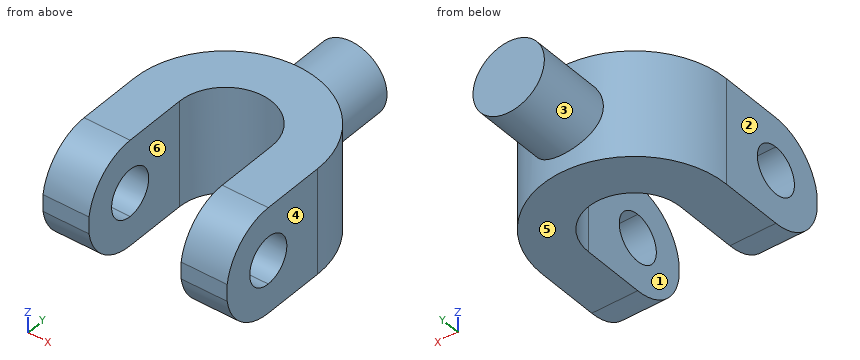
```python
from build123d import *

# Parameters (mm, degrees)
BOSS_EXTRUDE1_DEPTH = 29.21
CUT_EXTRUDE1_DEPTH  = 143.460247374


with BuildPart() as part:
    # Sketch1 → Boss-Extrude1 (new, symmetric)
    with BuildSketch(Plane.XY):
        with BuildLine():
            ThreePointArc((-152.609053498, 7.264609053), (-101.809053498, 58.064609053), (-51.009053498, 7.264609053))
            Line((-51.009053498, 7.264609053), (-51.009053498, -56.235390947))
            Line((-51.009053498, -56.235390947), (-76.409053498, -56.235390947))
            Line((-76.409053498, -56.235390947), (-76.409053498, 7.264609053))
            ThreePointArc((-76.409053498, 7.264609053), (-101.809053498, 32.664609053), (-127.209053498, 7.264609053))
            Line((-127.209053498, 7.264609053), (-127.209053498, -56.235390947))
            Line((-127.209053498, -56.235390947), (-152.609053498, -56.235390947))
            Line((-152.609053498, -56.235390947), (-152.609053498, 7.264609053))
        make_face()
    extrude(amount=BOSS_EXTRUDE1_DEPTH, both=True)

    # Sketch1<4> → Revolve1 (revolve)
    with BuildSketch(Plane.XY, mode=Mode.PRIVATE) as revolve1_sk:
        with BuildLine():
            Line((-121.502148415, 95.494177501), (-121.502148415, 54.092186533))
            ThreePointArc((-121.502148415, 54.092186533), (-111.853929407, 57.061601613), (-101.809053498, 58.064609053))
            Line((-101.809053498, 58.064609053), (-101.809053498, 95.494177501))
            Line((-101.809053498, 95.494177501), (-121.502148415, 95.494177501))
        make_face()
    revolve(revolve1_sk.sketch.rotate(Axis((-101.809053498, 95.494177501, 0), (0, -1, 0)), 270), axis=Axis((-101.809053498, 95.494177501, 0), (0, -1, 0)))

    # Sketch3 → Cut-Extrude1 (cut, through all)
    with BuildSketch(Plane(origin=(-51.009053498, 0, 0), x_dir=(0, 0, -1), z_dir=(1, 0, 0))):
        with BuildLine():
            ThreePointArc((-13.016901543, -27.398347302), (0, -40.415248845), (13.016901543, -27.398347302))
            Line((13.016901543, -27.398347302), (-13.016901543, -27.398347302))
        make_face()
        with BuildLine():
            Line((-13.016901543, -27.398347302), (13.016901543, -27.398347302))
            ThreePointArc((13.016901543, -27.398347302), (0, -14.381445758), (-13.016901543, -27.398347302))
        make_face()
        with BuildLine():
            ThreePointArc((-4.652850075, -56.235390947), (-22.238860702, -46.336593647), (-29.21, -27.398347302))
            Line((-29.21, -27.398347302), (-29.21, -56.235390947))
            Line((-29.21, -56.235390947), (-4.652850075, -56.235390947))
        make_face()
        with BuildLine():
            Line((29.21, -56.235390947), (29.21, -27.398347302))
            ThreePointArc((29.21, -27.398347302), (22.238860702, -46.336593647), (4.652850075, -56.235390947))
            Line((4.652850075, -56.235390947), (29.21, -56.235390947))
        make_face()
    extrude(amount=-CUT_EXTRUDE1_DEPTH, mode=Mode.SUBTRACT)


solid = part.part
```
Geometry check sheet. Reference: the model listing, model coordinates, mm. Face numbers are marked on the shaded views. A direction names the side the tool comes from. Coordinates: 2 decimals unless noted, no trailing zeros. Write each loop counter-clockwise with the first axis right and the second up, starting at its lowest first coordinate (ties: lowest second). Pieces come first, ordered by that corner, then holes. Notation, with made-up numbers: M 75.5,-4 L 130.5,-4 A19 cw 130.5,24 Z; hole C -3,81.5 d6. An arc over 180 degrees is marked long. Use one line per item in the form item = value. Start each with the question number.
1) Section check D-D on z = 8. Enter the section's corners in (x, y), and give its area (3 significant figures).
2) Thickness scan on probe 1 along X at (y, z) = (-11.5, 15.5); probe 2 along Z at (x, y) = (-65, -38); probe 3 along Y at (x, z) = (-147, 1.5). Record the ranges inside material, lowest first. Write a range as from..to.
3) Release check for a two-part mould opening along X. For the marked faces 3, 4, 5 and 6 record: pulls with the +X half, pulls with the -X half, needs draft (parallel to the pull), parting line crosses it, or undercut.
4) Section check A-A on z = 0. Enter the section's corners in (x, y).
5) Set-up check for the marked faces 1 and 2: record each of +Z, -Z, +X, -X, +Y, -Y from which the full face is reachable in a straight line by a thin tool's end or side.
6) Go/stop test with flat-tipped pins: pin 1 Ø8 at (y, z) = (48, 20.5) entering from -X; pin 2 Ø5 at (x, z) = (-136.5, 23) entering from +Y; pin 3 Ø8 at (x, z) = (-94, -8) entering from -Y. Record where each tip stops, or that it passes through.
7) Section check C-C on x = -143.5. Enter the section's corners in (y, z).
8) Section check B-B on y = -32. Enter the section's corners in (x, z).
Responses:
q1.outline = M -152.61,-55.49 L -127.21,-55.49 L -127.21,-37.67 L -152.61,-37.67 Z; M -152.61,-17.13 L -127.21,-17.13 L -127.21,7.26 A25.4 cw -76.41,7.26 L -76.41,-17.13 L -51.01,-17.13 L -51.01,7.26 A50.8 ccw -83.81,54.77 L -83.81,95.49 L -119.8,95.49 L -119.8,54.77 A50.8 ccw -152.61,7.26 Z; M -76.41,-55.49 L -51.01,-55.49 L -51.01,-37.67 L -76.41,-37.67 Z
q1.area = 6,570 mm2
q2.probe_1 = -152.61..-127.21, -76.41..-51.01
q2.probe_2 = -27.22..-7.55, 7.55..27.22
q2.probe_3 = -56.24..-40.33, -14.47..30.47
q3.face_3 = parting line crosses it
q3.face_4 = pulls with the +X half
q3.face_5 = needs draft
q3.face_6 = undercut
q4.outline = M -152.61,-56.24 L -127.21,-56.24 L -127.21,-40.42 L -152.61,-40.42 Z; M -152.61,-14.38 L -127.21,-14.38 L -127.21,7.26 A25.4 cw -76.41,7.26 L -76.41,-14.38 L -51.01,-14.38 L -51.01,7.26 A50.8 ccw -82.12,54.09 L -82.12,95.49 L -121.5,95.49 L -121.5,54.09 A50.8 ccw -152.61,7.26 Z; M -76.41,-56.24 L -51.01,-56.24 L -51.01,-40.42 L -76.41,-40.42 Z
q5.face_1 = +Z, -Z, -Y
q5.face_2 = +Z, -Z, -X, +Y, -Y
q6.pin_1 = -136.9
q6.pin_2 = 46.56
q6.pin_3 = 29.75
q7.outline = M -56.24,-4.65 A29.21 ccw -27.4,-29.21 L 36.29,-29.21 L 36.29,29.21 L -27.4,29.21 A29.21 ccw -56.24,4.65 Z; hole C -27.4,0 d26.03
q8.outline = M -152.61,-28.85 L -127.21,-28.85 L -127.21,-12.18 L -152.61,-12.18 Z; M -152.61,12.18 L -127.21,12.18 L -127.21,28.85 L -152.61,28.85 Z; M -76.41,-28.85 L -51.01,-28.85 L -51.01,-12.18 L -76.41,-12.18 Z; M -76.41,12.18 L -51.01,12.18 L -51.01,28.85 L -76.41,28.85 Z
